Build history of the part. All positions in model axes, mm. Face numbers are marked on the shaded views. A direction names the side the tool comes from. Round coordinates to 2 decimals unless told otherwise and drop trailing zeros. Write each loop counter-clockwise with the first axis right and the second up, starting at its lowest first coordinate (ties: lowest second). Pieces come first, ordered by that corner, then holes.
Item 1: Band-saw the part on C-C, the plane x = -3.5. Write the cut outline in (y, z), then the cut area to 3 significant figures.
Item 2: Band-saw the part on D-D, the plane z = -10. Write the cut outline in (x, y).
Item 3: Wall check: probe 1 along X at (y, z) = (13.75, -2); probe 2 along Y at (x, z) = (3, 7); probe 3 along Y at (x, z) = (-19.5, 5). Give the ranges that are in metal, low to high.
Item 4: Drop flat-ended pins along their axis: pin 1 Ø3 at (x, y) = (-3, 11.5) entering from +Z; pin 2 Ø4 at (x, y) = (-6.5, 15.5) entering from -Z; pin 3 Ø2 at (x, z) = (-13, 3) entering from -Y. Give the stop position or say it passes through.
Item 5: 3-axis set-ups, long thin cutter, end or side, ignore diameter. For the marked faces 1, 2, 3, 4 and 5: which of +Z, -Z, +X, -X, +Y, -Y reach the whole face in a straight line?
Item 6: Band-saw the part on A-A, the plane y = 16. Write the cut outline in (x, z), then the cut area to 3 significant figures.
Item 7: Mould opens along X. For the marked faces 6, 7 and 8 say: +X half, -X half, draft (parallel to the pull), parting line (faces both ways), or undercut.
Item 8: Band-saw the part on B-B, the plane z = 2.5. Write the cut outline in (x, y), then the cut area to 3 significant figures.
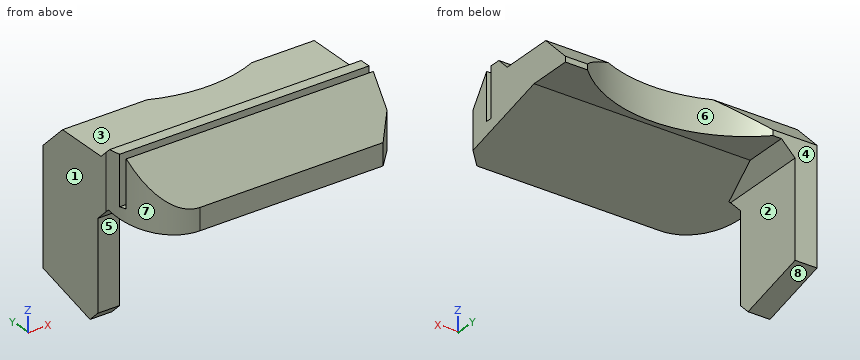
```python
from build123d import *
from OCP.BRepFilletAPI import BRepFilletAPI_MakeChamfer

# Parameters (mm, degrees)
BOSS_EXTRUDE1_DEPTH  = 21
BOSS_EXTRUDE4_DEPTH  = 6
CHAMFER4_SIZE        = 5
BOSS_EXTRUDE5_DEPTH  = 4
BOSS_EXTRUDE10_DEPTH = 4
FILLET1_R            = 10
CHAMFER5_SIZE        = 2.5
CHAMFER5_SIZE2       = 2.041241452


with BuildPart() as part:
    # Sketch1 → Boss-Extrude1 (new, symmetric)
    with BuildSketch(Plane(origin=(0, 0, 0), x_dir=(0, 0, -1), z_dir=(1, 0, 0))):
        Polygon((0, -6), (4, -6), (-0.849880383, 12.1), (-6.849880383, 12.1), (-6.849880383, 5.250119617), (-9, 3.1), (-9, 1.1), (0, 1.1), (0, 0), (-8.56888804, 0), align=None)
    extrude(amount=BOSS_EXTRUDE1_DEPTH, both=True)

    # Sketch7 → Boss-Extrude4 (add)
    with BuildSketch(Plane.XY.offset(6.849880383)):
        with BuildLine():
            Line((-21, 12.1), (-21, 20.1))
            Line((-21, 20.1), (-16.941074346, 20.1))
            ThreePointArc((-16.941074346, 20.1), (0, 13.1), (16.941074346, 20.1))
            Line((16.941074346, 20.1), (21, 20.1))
            Line((21, 20.1), (21, 12.1))
            Line((21, 12.1), (-21, 12.1))
        make_face()
    extrude(amount=-BOSS_EXTRUDE4_DEPTH)

    # Chamfer4
    chamfer4_edges = [part.edges().sort_by_distance(p)[0] for p in [
        (-18.970537173, 20.1, 6.849880383),
        (18.970537173, 20.1, 6.849880383),
    ]]
    chamfer(chamfer4_edges, length=CHAMFER4_SIZE)

    # Sketch15 → Boss-Extrude5 (add)
    with BuildSketch(Plane.ZY.offset(21)):
        Polygon((9, 1.1), (9, 3.1), (6.849880383, 5.250119617), (6.849880383, 15.1), (1.849880383, 20.1), (0.849880383, 20.1), (0.849880383, 12.1), (-4, -6), (0, -6), (8.56888804, 0), (0, 0), (0, 1.1), align=None)
    extrude(amount=BOSS_EXTRUDE5_DEPTH)

    # Sketch22 → Boss-Extrude10 (add)
    with BuildSketch(Plane.ZY.offset(25)):
        Polygon((0.849880383, 6.1), (0.849880383, 1.1), (-4.150119617, 6.1), (-19.150119617, 6.1), (-22.901408311, 6.1), (-19.150119617, 20.1), (0.849880383, 20.1), align=None)
    extrude(amount=-BOSS_EXTRUDE10_DEPTH)

    # Fillet1
    # the kernel refuses this fillet: 10 mm, written as the material it takes off along each edge
    with BuildSketch(Plane(origin=(-25, -6, -29), x_dir=(1, 0, 0), z_dir=(0, 0, 1))) as fillet1_piece_1:
        with BuildLine():
            CenterArc((FILLET1_R, FILLET1_R), FILLET1_R, 180, 90)
            Line((0, FILLET1_R), (0, 0))
            Line((0, 0), (FILLET1_R, 0))
        make_face()
    extrude(amount=54, mode=Mode.SUBTRACT)

    # Chamfer5: one chamfer whose edges measure the first distance from different faces: ONE call of the kernel's chamfer builder (chamfer() names one face for all edges)
    chamfer5_edges_1 = [part.edges().sort_by_distance(p)[0] for p in [
        (21, -6, -2),
        (-21, 16.1, 0.849880383),
    ]]
    chamfer5_edges_2 = [part.edges().sort_by_distance(p)[0] for p in [
        (-23, 6.1, -22.901408311),
    ]]
    chamfer5_side_2 = [part.faces().sort_by_distance(p)[0] for p in [
        (-23, 6.1, -13.525763964),
    ]]
    chamfer5 = BRepFilletAPI_MakeChamfer(part.part.solid().wrapped)
    for e in chamfer5_edges_1:
        chamfer5.Add(CHAMFER5_SIZE, e.wrapped)
    for e in chamfer5_edges_2:
        chamfer5.Add(CHAMFER5_SIZE, CHAMFER5_SIZE2, e.wrapped, chamfer5_side_2[0].wrapped)  # the first distance lies on this face
    add(Compound.cast(chamfer5.Shape()), mode=Mode.REPLACE)


solid = part.part
```
Results:
1. outline: (-6, -4) - (12.1, 0.85) - (13.36, 0.85) - (13.36, 6.85) - (5.25, 6.85) - (3.1, 9) - (1.1, 9) - (1.1, 0) - (0, 0) - (0, 8.57) - (-6, 0) - close
1. area: 144 mm2
2. outline: (-25, 6.1) - (-21, 6.1) - (-21, 20.1) - (-25, 20.1) - close
3. probe 1: x = -25 to -21
3. probe 2: y = -1.1 to 0, 1.1 to 5.1
3. probe 3: y = -2.5 to 0, 1.1 to 16.95
4. pin 1: stops at z = 6.85
4. pin 2: stops at z = 0.85
4. pin 3: stops at y = -4.6
5. face 1: +Z, -Z, -X, +Y, -Y
5. face 2: -Z, +X, +Y
5. face 3: +Z, +X, -X, +Y
5. face 4: +Z, -Z, +X, -X, +Y
5. face 5: -Z, +X, -X, -Y
6. outline: (-25, -20.25) - (-21, -20.25) - (-21, -1.65) - (-18.5, 0.85) - (-11.44, 0.85) - (-11.44, 5.95) - (-25, 5.95) - close; (11.44, 0.85) - (21, 0.85) - (21, 5.95) - (11.44, 5.95) - close
6. area: 205 mm2
7. face 6: undercut
7. face 7: -X half
7. face 8: draft
8. outline: (-25, 4) arc R10 ccw to (-24.57, 1.1) - (21, 1.1) - (21, 19.45) - (16.26, 19.45) arc R24 cw to (-16.26, 19.45) - (-25, 19.45) - close; (-24.17, 0) arc R10 ccw to (-20.65, -4.25) - (20.25, -4.25) - (21, -3.5) - (21, 0) - close
8. area: 887 mm2
